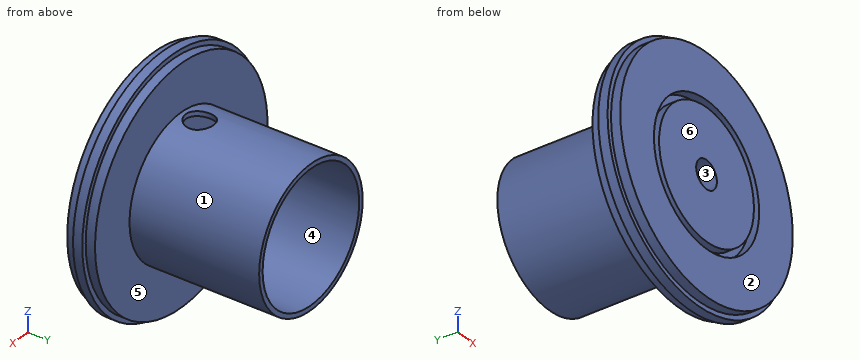
Autodesk Inventor part; units mm, degrees
ref_plane "YZ Plane" through (0, 0, 0) normal (1, 0, 0) x (0, 1, 0)
ref_plane "XZ Plane" through (0, 0, 0) normal (0, 1, 0) x (-1, 0, 0)
ref_plane "XY Plane" through (0, 0, 0) normal (0, 0, 1) x (1, 0, 0)
sketch "Sketch1" plane through (0, 0, 0) normal (0, 1, 0) x (-1, 0, 0)
  circle A0 centre (0, 0) radius 25
  dimension "d0" = 50
extrude "Extrusion1" add sketch "Sketch1" along normal blind 2
sketch "Sketch2" plane through (0, 2, 0) normal (0, 1, 0) x (1, 0, 0)
  circle A0 centre (0, 0) radius 26
  dimension "d3" = 52
extrude "Extrusion2" add sketch "Sketch2" along normal blind 2
sketch "Sketch6" plane through (0, 4, 0) normal (0, 1, 0) x (1, 0, 0)
  circle A0 centre (0, 0) radius 25
  dimension "d17" = 50
extrude "Extrusion6" add sketch "Sketch6" along normal blind 2
sketch "Sketch3" plane through (0, 4, 0) normal (0, 1, 0) x (1, 0, 0)
  circle A0 centre (0, 0) radius 15
  circle A1 centre (0, 0) radius 14
  dimension "d6" = 30
  dimension "d7" = 28
extrude "Extrusion3" add sketch "Sketch3" along normal blind 30
sketch "Sketch5" plane through (0, 0, 0) normal (0, 0, 1) x (1, 0, 0)
  circle A0 centre (0, 10) radius 3
  line L0 (26, 4) -> (-26, 4)
  point P0 (0, 0)
  dimension "d13" = 6
  dimension "d14" = 6
extrude "Extrusion5" cut sketch "Sketch5" along normal blind 30
sketch "Sketch7" plane through (0, 6, 0) normal (0, 1, 0) x (1, 0, 0)
  circle A0 centre (0, 0) radius 3
  dimension "d20" = 6
extrude "Extrusion7" cut sketch "Sketch7" against normal through all
sketch "Sketch8" plane through (0, 0, 0) normal (0, -1, 0) x (1, 0, 0)
  circle A0 centre (0, 0) radius 3
  circle A1 centre (0, 0) radius 13.75
  circle A2 centre (0, 0) radius 15.25
  dimension "d23" = 27.5
  dimension "d24" = 30.5
extrude "Extrusion8" cut sketch "Sketch8" against normal blind 2 contours A2
properties part number "Stack-lens holder"
For this review, take the finished solid that the model builds, in its own axes (mm). Face numbers are marked on the shaded views. A direction names the side the tool comes from. Give positions to 0.01 mm unless a question says otherwise; leave off trailing zeros. Order: outer loops, then holes, each group sorted by start corner. A loop starts at its lowest first (then second) coordinate and runs counter-clockwise, first axis right, second up. Notation, with made-up numbers: M 65.5,43.5 L 94.5,43.5 A33 cw 94.5,71.5 Z; hole C -13.75,-8.75 d6. An arc over 180 degrees is marked long. Answer in a Markdown table with one row per item. Add a question column.
(1) Consider section D-D on z = 22.5. State the section outline as (x, y) points, and give its area (3 significant figures).
(2) For pin 1 (8 mm diameter, centred on x = -8.5, z = 1.5, fed in from +Y); pin 2 (10 mm diameter, centred on x = -3, y = 28.5, fed in from -Z); pin 3 (2 mm diameter, centred on x = -3, y = 19, fed in from -Z), all flat-tipped, find the tip position at first contact; note any pin that passes through.
(3) Wall thickness on probe 1 along Z at (x, y) = (0, 1); probe 2 along X at (y, z) = (3, 0); probe 3 along X at (y, z) = (18.75, 0): over which ranges is each line inside the solid? List them lowest first. Write a range as [from, to].
(4) Consider section C-C on y = 31. State the section outline as (x, z) points, and give its area (3 significant figures).
(5) For the marked faces 5 and 6, list the 3-axis set-ups (+Z, -Z, +X, -X, +Y, -Y) from which the entire face can be reached by the end or side of a thin tool; tool diameter is ignored.
(6) Mouldability with a two-part tool opening along X and no side actions: class the marked faces 1, 2, 3 and 4 as +X half, -X half, draft (parallel to the pull), parting line (faces both ways), or undercut.
(7) Consider section B-B on x = 0. Give the number of separate pieces and of enclosed holes in the cut face, and give its area (3 significant figures).
Evaluation:
| question | item | result |
|---|---|---|
| 1 | outline | M -13.03,2 L -10.9,2 L -10.9,0 L 10.9,0 L 10.9,2 L 13.03,2 L 13.03,4 L 10.9,4 L 10.9,6 L -10.9,6 L -10.9,4 L -13.03,4 Z |
| 1 | area | 139 mm^2 |
| 2 | pin 1 | stops at y = 6 |
| 2 | pin 2 | stops at z = -15 |
| 2 | pin 3 | stops at z = -14.87 |
| 3 | probe 1 | z = [-25, -15.25], [-13.75, -3], [3, 13.75], [15.25, 25] |
| 3 | probe 2 | x = [-26, -3], [3, 26] |
| 3 | probe 3 | x = [-15, -14], [14, 15] |
| 4 | outline | C 0,0 d30; hole C 0,0 d28 |
| 4 | area | 91.1 mm^2 |
| 5 | face 5 | +Y |
| 5 | face 6 | +Z, -Z, +X, -X, -Y |
| 6 | face 1 | parting line |
| 6 | face 2 | draft |
| 6 | face 3 | undercut |
| 6 | face 4 | undercut |
| 7 | separate pieces | 3 |
| 7 | enclosed holes | 0 |
| 7 | area | 312 mm^2 |
